The model under review builds one solid part; all positions refer to its coordinate system, in mm. A direction names the side the tool comes from. Coordinates: 2 decimals unless noted, no trailing zeros. Loops run counter-clockwise (first coordinate to the right, second up) from the corner with the lowest first, then second, coordinate; pieces in that order, holes last. Notation, with made-up numbers: M 2,-21 L 42,-21 A13 cw 42,-12 Z; hole C -21.75,-35 d4. An arc over 180 degrees is marked long. Use CSV: the item, a comma, the result in double quotes. Start each with the question number.
1. For L1, parallel to X at y = 2, z = 80; L2, parallel to Z at x = 33, y = 1.3; L3, parallel to Z at x = 181.5, y = 2.05, list the stretches that pass through material, from the lowest coordinate up.
2. Tool access review of faces 5 (the flat face through (-6.254, 2, -46)), 6 (the flat face through (-29, 2, -38.535)), 7 (the flat face through (206, 2, 16.465)): name each direction out of +Z, -Z, +X, -X, +Y, -Y from which nothing blocks a thin tool from reaching the whole face with its end or side.
3. Draft analysis for pull direction X (two halves, no side actions). For faces 1 (the flat face through (98.746, 2, -46)), 2 (the flat face through (206, 2, -43.535)), 3 (the flat face through (-36.254, 2, -44)), 4 (the flat face through (173.746, 2, -46)), state which applies: +X half, -X half, draft (parallel to the pull), parting line (faces both ways), or undercut.
4. Add section C-C, the plane y = 3.85. Write out the cut boundary in (x, z).
5. Clearance check with flat-ended pins moving along their axes: P1, Ø1.5, axis at x = 207, y = 2, coming from the -Z side; P2, Ø8, axis at x = 162.5, z = 80.5, coming from the -Y side; P3, Ø1.5, axis at y = 4, z = 56.5, coming from the +X side. State where each tip first meets the part, or that it passes through.
6. Add section D-D, the plane z = 28. Write out the cut boundary in (x, y), then the cut area to 4 significant figures.
7. Add section B-B, the plane x = 73. Write out the cut boundary in (y, z), then the cut area to 3 significant figures.
from build123d import *

# Parameters (mm, degrees)
SKETCH_1_W          = 5
SKETCH_1_H          = 60
SKETCH_1_W_2        = 30
SKETCH_1_H_2        = 5
SKETCH_1_W_3        = 15
EXTRUDE_1_DEPTH     = 5
FILLET_1_R          = 5
SKETCH_2_W          = 239.490005879
SKETCH_2_H          = 213.108485662
CUT_EXTRUDE_2_DEPTH = 10
SKETCH_3_W          = 110
SKETCH_3_H          = 2.5
SKETCH_3_W_2        = 115
CUT_EXTRUDE_3_DEPTH = 10
SKETCH_4_W          = 5
SKETCH_4_H          = 5
CUT_EXTRUDE_4_DEPTH = 5


with BuildPart() as part:
    # 草圖1 → 填料-伸長1 (new body)
    with BuildSketch(Plane(origin=(0, 0, 0), x_dir=(1, 0, 0), z_dir=(0, 1, 0))):
        Polygon((198.746286718, -286.464902661), (198.746286718, -256.464902661), (183.246286718, -256.464902661), (183.246286718, -266.464902661), (124.746286718, -266.464902661), (124.746286718, -262.464902661), (109.246286718, -262.464902661), (109.246286718, -266.464902661), (-21.253713282, -266.464902661), (-21.253713282, 38.535097339), (-36.253713282, 38.535097339), (-36.253713282, 43.535097339), (203.746286718, 43.535097339), (203.746286718, -286.464902661), align=None)
        with Locations((206.246286718, -256.464902661)):
            Rectangle(SKETCH_1_W, SKETCH_1_H)
        with Locations((206.246286718, 13.535097339)):
            Rectangle(SKETCH_1_W, SKETCH_1_H)
        with Locations((188.746286718, 46.035097339)):
            Rectangle(SKETCH_1_W_2, SKETCH_1_H_2)
        with Locations((-21.253713282, 46.035097339)):
            Rectangle(SKETCH_1_W_2, SKETCH_1_H_2)
        with Locations((91.246286718, 46.035097339)):
            Rectangle(SKETCH_1_W_3, SKETCH_1_H_2)
        with Locations((76.246286718, 46.035097339)):
            Rectangle(SKETCH_1_W_3, SKETCH_1_H_2)
        with Locations((206.246286718, -166.464902661)):
            Rectangle(SKETCH_1_W, SKETCH_1_H)
        with Locations((206.246286718, -76.464902661)):
            Rectangle(SKETCH_1_W, SKETCH_1_H)
    extrude(amount=EXTRUDE_1_DEPTH)

    # 圓角1
    fillet_1_edges = [part.edges().sort_by_distance(p)[0] for p in [
        (208.746286718, 5, -13.535097339),
        (208.746286718, 5, 76.464902661),
        (208.746286718, 5, 166.464902661),
        (208.746286718, 5, 256.464902661),
    ]]
    fillet(fillet_1_edges, radius=FILLET_1_R - 0.0001)  # a hair under: the kernel refuses the full size

    # 草圖2 → 除料-伸長2 (cut)
    with BuildSketch(Plane(origin=(0, 5, 0), x_dir=(1, 0, 0), z_dir=(0, 1, 0))):
        with Locations((89.001283779, -193.019145492)):
            Rectangle(SKETCH_2_W, SKETCH_2_H)
    extrude(amount=-CUT_EXTRUDE_2_DEPTH, mode=Mode.SUBTRACT)

    # 草圖3 → 除料-伸長3 (cut)
    with BuildSketch(Plane.XY.offset(86.464902661)):
        with Locations((33.746286718, 3.75)):
            Rectangle(SKETCH_3_W, SKETCH_3_H)
        with Locations((151.246286718, 1.25)):
            Rectangle(SKETCH_3_W_2, SKETCH_3_H)
    extrude(amount=-CUT_EXTRUDE_3_DEPTH, mode=Mode.SUBTRACT)

    # 草圖4 → 除料-伸長4 (cut)
    with BuildSketch(Plane.XY.offset(86.464902661)):
        with Locations((91.246286718, 2.5)):
            Rectangle(SKETCH_4_W, SKETCH_4_H)
    extrude(amount=-CUT_EXTRUDE_4_DEPTH, mode=Mode.SUBTRACT)


solid = part.part
Computed:
1,L1,"x = -21.25 to 93.75"
1,L2,"z = -43.54 to 86.46"
1,L3,"z = -48.54 to 76.46"
2,face 5,"-Z, +Y, -Y"
2,face 6,"+Z, -X, +Y, -Y"
2,face 7,"+X, +Y, -Y"
3,face 1,"undercut"
3,face 2,"draft"
3,face 3,"-X half"
3,face 4,"undercut"
4,outline,"M -36.25,-48.54 L -6.25,-48.54 L -6.25,-43.54 L 68.75,-43.54 L 68.75,-48.54 L 98.75,-48.54 L 98.75,-43.54 L 173.75,-43.54 L 173.75,-48.54 L 203.75,-48.54 L 203.75,-43.54 L 206.94,-43.54 L 206.94,16.46 L 203.75,16.46 L 203.75,46.46 L 206.94,46.46 L 206.94,86.46 L 93.75,86.46 L 93.75,81.46 L 88.75,81.46 L 88.75,76.46 L -21.25,76.46 L -21.25,-38.54 L -36.25,-38.54 Z"
5,P1,"stops at z = -43.54"
5,P2,"stops at y = 2.5"
5,P3,"stops at x = 207.55"
6,outline,"M -21.25,0 L 203.75,0 L 203.75,5 L -21.25,5 Z"
6,area,"1,125 mm^2"
7,outline,"M 0,-48.54 L 5,-48.54 L 5,76.46 L 2.5,76.46 L 2.5,86.46 L 0,86.46 Z"
7,area,"650 mm^2"
